Model file for the job. Use its own axes, mm. Round coordinates to 2 decimals unless told otherwise and drop trailing zeros. Loops run counter-clockwise (first coordinate to the right, second up) from the corner with the lowest first, then second, coordinate; pieces in that order, holes last. Notation, with made-up numbers: (-5.5, 27) - (9.5, 27) arc R24 cw to (9.5, 55) - close; hole circle Ø3 at (-1.5, 8.25). An arc over 180 degrees is marked (long way). Answer as a JSON object with one key per item and string values.
Autodesk Inventor part; units mm, degrees
ref_plane "YZ Plane" through (0, 0, 0) normal (1, 0, 0) x (0, 1, 0)
ref_plane "XZ Plane" through (0, 0, 0) normal (0, 1, 0) x (-1, 0, 0)
ref_plane "XY Plane" through (0, 0, 0) normal (0, 0, 1) x (1, 0, 0)
sketch "Sketch1" plane through (0, 0, 0) normal (1, 0, 0) x (0, 1, 0)
  circle A0 centre (0, 0) radius 12
  circle A1 centre (0, 0) radius 17.5
  line L0 (0, 0) -> (0, -201.7) construction
  line L1 (-17.5, 0) -> (-17.5, -201.7)
  line L2 (17.5, -201.7) -> (17.5, 0)
  arc A2 (17.5, 0) -> (-17.5, 0) centre (0, 0) ccw
  arc A3 (-17.5, -201.7) -> (17.5, -201.7) centre (0, -201.7) ccw
  line L3 (0, 0) -> (201.7, 0) construction
  circle A4 centre (0, -60.425) radius 2.75
  circle A5 centre (0, -120.85) radius 2.75
  circle A6 centre (0, -181.275) radius 2.75
  circle A7 centre (0, -201.7) radius 4.5
  circle A8 centre (0, 50) radius 2.75
  arc A9 (7.3485, 51.5) -> (-7.3485, 51.5) centre (0, 50) ccw
  line L4 (7.3485, 51.5) -> (17.1464, 3.5)
  line L5 (-7.3485, 51.5) -> (-17.1464, 3.5)
  arc A10 (17.1464, 3.5) -> (-17.1464, 3.5) centre (0, 0) ccw
  point P0 (0, -100.85)
  dimension "d0" = 24
  dimension "d1" = 35
  dimension "d7" = 201.7
  dimension "d8" = 90
  dimension "d9" = 35
  dimension "d13" = 5.5
  dimension "d14" = 60.425
  dimension "d15" = 17.5
  dimension "d18" = 60.425
  dimension "d23" = 9
  dimension "d24" = 5.5
  dimension "d25" = 17.5
  dimension "d26" = 50
  dimension "d27" = 15
extrude "Extrusion1" add sketch "Sketch1" along normal blind 5 contours A1 | L2 A3 L1 A1 | A1 L5 A9 L4 | A8
sketch "Sketch2" plane through (5, 0, 0) normal (1, 0, 0) x (0, 0, -1)
  circle A0 centre (0, 0) radius 13.5
  dimension "d4" = 27
extrude "Extrusion2" cut sketch "Sketch2" against normal blind 1.1
sketch "Sketch4" plane through (0, 0, 0) normal (-1, 0, 0) x (0, 0, 1)
  circle A0 centre (50, 0) radius 2.75
  arc A1 (51.5, -7.3485) -> (51.5, 7.3485) centre (50, 0) ccw
  point P0 (0, 0)
  dimension "d28" = 5.5
extrude "Extrusion4" cut sketch "Sketch4" against normal blind 10
properties part number "Bearing Holder" material "Aluminum 6061"
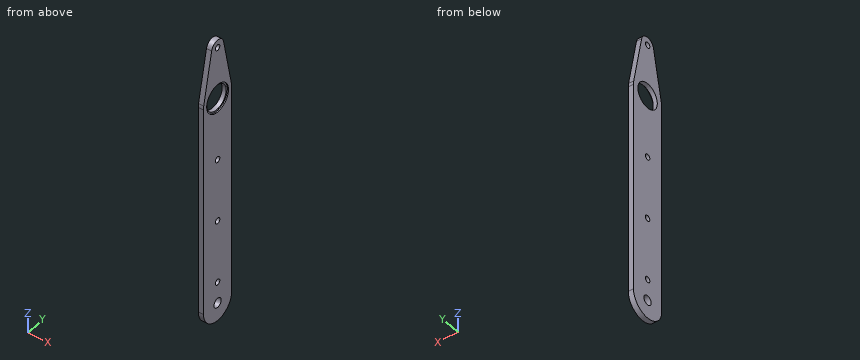
1) Slice it at A-A on z = -120.85. List the corners of the cut face in (x, y).
Values follow:
{"outline": "(0, -17.5) - (5, -17.5) - (5, -2.75) - (0, -2.75) - close; (0, 2.75) - (5, 2.75) - (5, 17.5) - (0, 17.5) - close"}
2) Drop flat-ended pins along their axis: P1, Ø2, axis at x = 3, y = -4.5, coming from the -Z side; P2, Ø3, axis at x = 0.5, y = 2, coming from the -Z side. Give the stop position or say it passes through.
Values follow:
{"P1": "z = -218.85", "P2": "z = -219.19"}
3) Probe probe 1 along Z at (x, y) = (3.75, 4); probe 2 along Y at (x, z) = (1.2, -0.5); probe 3 along Y at (x, z) = (1.3, 50). List the from-to ranges inside material, lowest first.
Values follow:
{"probe 1": "-218.74 to -203.76, -199.64 to -11.31, 11.31 to 56.34", "probe 2": "-17.5 to -11.99, 11.99 to 17.5", "probe 3": "-7.65 to -2.75, 2.75 to 7.65"}
4) Slice it at B-B on y = 0. Count the separate pieces of the cut face and the enclosed holes in it, then the cut area to 3 significant figures.
Values follow:
{"separate pieces": "7", "enclosed holes": "0", "area": "1,110 mm²"}
